from build123d import *

# Parameters (mm, degrees)
BOSS_EXTRUDE1_DEPTH  = 20
SKETCH2_W            = 14
SKETCH2_H            = 4
CUT_EXTRUDE1_DEPTH   = 3
SKETCH4_R            = 1.1
CUT_EXTRUDE2_DEPTH   = 20
SKETCH3_R            = 1.25
SKETCH3_R_2          = 1.1
CUT_EXTRUDE3_DEPTH   = 2
SKETCH9_W            = 10.2
SKETCH9_H            = 1
BOSS_EXTRUDE11_DEPTH = 10


with BuildPart() as part:
    # Sketch1 → Boss-Extrude1 (new body)
    with BuildSketch(Plane.XY):
        Polygon((0, 11), (0, -8), (20, -8), (20, -6), (10.2, -6), (10.2, 11), (8.2, 11), (8.2, 2), (7.2, 2), (7.2, -6), (3, -6), (3, 2), (2, 2), (2, 11), align=None)
    extrude(amount=BOSS_EXTRUDE1_DEPTH)

    # Sketch2 → Cut-Extrude1 (cut)
    with BuildSketch(Plane.ZY):
        with Locations((10, -4)):
            Rectangle(SKETCH2_W, SKETCH2_H)
    extrude(amount=-CUT_EXTRUDE1_DEPTH, mode=Mode.SUBTRACT)

    # Sketch4 → Cut-Extrude2 (cut)
    with BuildSketch(Plane(origin=(0, -6, 0), x_dir=(1, 0, 0), z_dir=(0, 1, 0))):
        with Locations(Location((15.5, -5, 0), (0, 0, 270))):
            Circle(SKETCH4_R)
        with Locations(Location((15.5, -15, 0), (0, 0, 270))):
            Circle(SKETCH4_R)
    extrude(amount=-CUT_EXTRUDE2_DEPTH, mode=Mode.SUBTRACT)

    # Sketch3 → Cut-Extrude3 (cut)
    with BuildSketch(Plane(origin=(10.2, 0, 0), x_dir=(0, 0, -1), z_dir=(1, 0, 0))):
        with Locations((-15.421154519, 6.5)):
            Circle(SKETCH3_R)
        with Locations((-5.315777108, 6.5)):
            Circle(SKETCH3_R_2)
    extrude(amount=-CUT_EXTRUDE3_DEPTH, mode=Mode.SUBTRACT)

    # Sketch9 → Boss-Extrude11 (add)
    with BuildSketch(Plane(origin=(0, 11, 0), x_dir=(1, 0, 0), z_dir=(0, 1, 0))):
        with Locations((5.1, 0.5)):
            Rectangle(SKETCH9_W, SKETCH9_H)
        with Locations((5.1, -20.5)):
            Rectangle(SKETCH9_W, SKETCH9_H)
    extrude(amount=-BOSS_EXTRUDE11_DEPTH)


solid = part.part
Can you work these out from the model? Positions are in its coordinate system, mm. A direction names the side the tool comes from. Give positions to 0.01 mm unless a question says otherwise; leave off trailing zeros. Loops run counter-clockwise (first coordinate to the right, second up) from the corner with the lowest first, then second, coordinate; pieces in that order, holes last. Notation, with made-up numbers: (-11.75, 69.25) - (1.25, 69.25) arc R11 ccw to (1.25, 83.25) - close; hole circle Ø5 at (16.5, -5.5). An arc over 180 degrees is marked (long way). Answer as a JSON object with one key per item and string values.
Q1. Which directions (+Z, -Z, +X, -X, +Y, -Y) give clear straight access to the entire face, cutting with the end or side of a thin tool? Please do faces 5 (the flat face through (1, -2, 10)), 6 (the flat face through (3, 0, 10)), 7 (the flat face through (8, -4, 20)).
Geometry says:
{"face 5": "-X", "face 6": "+Y", "face 7": "+Z, +X, -X, -Y"}
Q2. Will these pins go through, and if not, where does the flat tip stop? P1, Ø0.9, axis at x = 1.5, y = -4.5, coming from the +Z side; P2, Ø4, axis at y = -3, z = 7, coming from the -X side; P3, Ø3, axis at y = 5.5, z = 2.5, coming from the +X side; P4, Ø2, axis at y = 6.5, z = 15.42, coming from the +X side.
Geometry says:
{"P1": "z = 20", "P2": "x = 0", "P3": "x = 10.2", "P4": "x = 2"}
Q3. If we mould it in two halves opening along X, with no side actions, what happens to faces 1 (the flat face through (0, 2, 10)), 2 (the flat face through (5, 1, -0.5)), 3 (the flat face through (2, 6, 10)), 4 (the flat face through (10.2, 3, 10))? For each: pulls with the +X half, pulls with the -X half, needs draft (parallel to the pull), parting line crosses it, or undercut.
Geometry says:
{"face 1": "pulls with the -X half", "face 2": "needs draft", "face 3": "undercut", "face 4": "pulls with the +X half"}
Q4. Imagine slicing it at D-D on y = 6.5. Write out the boundary of the cut face in (x, z), plus the area to 3 significant figures.
Geometry says:
{"outline": "(0, -1) - (10.2, -1) - (10.2, 4.22) - (8.2, 4.22) - (8.2, 0) - (2, 0) - (2, 20) - (8.2, 20) - (8.2, 16.67) - (10.2, 16.67) - (10.2, 21) - (0, 21) - close; (8.2, 6.42) - (10.2, 6.42) - (10.2, 14.17) - (8.2, 14.17) - close", "area": "91.0 mm²"}
Q5. Imagine slicing it at C-C on z = 5. Write out the boundary of the cut face in (x, y).
Geometry says:
{"outline": "(0, -8) - (14.4, -8) - (14.4, -6) - (10.2, -6) - (10.2, 5.45) - (8.2, 5.45) - (8.2, 2) - (7.2, 2) - (7.2, -6) - (0, -6) - close; (0, -2) - (3, -2) - (3, 2) - (2, 2) - (2, 11) - (0, 11) - close; (8.2, 7.55) - (10.2, 7.55) - (10.2, 11) - (8.2, 11) - close; (16.6, -8) - (20, -8) - (20, -6) - (16.6, -6) - close"}
Q6. Imagine slicing it at B-B on x = 15.5. Write out the boundary of the cut face in (y, z).
Geometry says:
{"outline": "(-8, 0) - (-6, 0) - (-6, 3.9) - (-8, 3.9) - close; (-8, 6.1) - (-6, 6.1) - (-6, 13.9) - (-8, 13.9) - close; (-8, 16.1) - (-6, 16.1) - (-6, 20) - (-8, 20) - close"}
Q7. Imagine slicing it at A-A on y = -2.75. Write out the boundary of the cut face in (x, z), plus the area to 3 significant figures.
Geometry says:
{"outline": "(0, 0) - (3, 0) - (3, 3) - (0, 3) - close; (0, 17) - (3, 17) - (3, 20) - (0, 20) - close; (7.2, 0) - (10.2, 0) - (10.2, 20) - (7.2, 20) - close", "area": "78.0 mm²"}
Q8. If I drill on L1, parallel to X at y = -2.75, z = 2.5; L2, parallel to Z at x = 5.25, y = 9.25; L3, parallel to Z at x = 15.75, y = -6.75, over which ranges is the centre line in solid material (lowest first)?
Geometry says:
{"L1": "0 to 3, 7.2 to 10.2", "L2": "-1 to 0, 20 to 21", "L3": "0 to 3.93, 6.07 to 13.93, 16.07 to 20"}
